Autodesk Inventor part; units mm, degrees
ref_plane "YZ Plane" through (0, 0, 0) normal (1, 0, 0) x (0, 1, 0)
ref_plane "XZ Plane" through (0, 0, 0) normal (0, 1, 0) x (-1, 0, 0)
ref_plane "XY Plane" through (0, 0, 0) normal (0, 0, 1) x (1, 0, 0)
sketch "草圖3" plane through (0, 0, 0) normal (0, 1, 0) x (-1, 0, 0)
  circle A0 centre (0, 0) radius 25
  circle A1 centre (0, 0) radius 70
  line L0 (5, 5) -> (61, 5)
  line L1 (61, 5) -> (61, 32.4)
  line L2 (61, 32.4) -> (5, 32.4)
  line L3 (5, 32.4) -> (5, 5)
  line L4 (19, 33.9) -> (12, 33.9)
  line L5 (12, 33.9) -> (12, 30.9)
  line L6 (12, 30.9) -> (19, 30.9)
  line L7 (19, 30.9) -> (19, 33.9)
  line L8 (54, 33.9) -> (47, 33.9)
  line L9 (47, 33.9) -> (47, 30.9)
  line L10 (47, 30.9) -> (54, 30.9)
  line L11 (54, 30.9) -> (54, 33.9)
  line L12 (61, 18.7) -> (5, 18.7)
  line L13 (19, 3.5) -> (12, 3.5)
  line L14 (12, 3.5) -> (12, 6.5)
  line L15 (12, 6.5) -> (19, 6.5)
  line L16 (19, 6.5) -> (19, 3.5)
  line L17 (54, 3.5) -> (47, 3.5)
  line L18 (47, 3.5) -> (47, 6.5)
  line L19 (47, 6.5) -> (54, 6.5)
  line L20 (54, 6.5) -> (54, 3.5)
  line L21 (0, 0) -> (55, 0)
  line L22 (19.1511, -16.0697) -> (42.1324, -35.3533)
  arc A2 (42.1324, -35.3533) -> (55, 0) centre (0, 0) ccw
  line L23 (0, 0) -> (15.7742, -52.6894)
  arc A3 (-21.7844, -50.5019) -> (15.7742, -52.6894) centre (0, 0) ccw
  line L24 (-9.902, -22.9554) -> (-21.7844, -50.5019)
  line L25 (0, 0) -> (-45.9518, -30.223)
  arc A4 (-54.6281, 6.3851) -> (-45.9518, -30.223) centre (0, 0) ccw
  line L26 (-24.831, 2.9023) -> (-54.6281, 6.3851)
  line L27 (0, 0) -> (-42.1324, 35.3533)
  arc A5 (-9.5506, 54.1644) -> (-42.1324, 35.3533) centre (0, 0) ccw
  line L28 (-4.3412, 24.6202) -> (-9.5506, 54.1644)
  line L29 (17.5, 0) -> (-21.7065, 0)
  line L30 (7.8968, 70) -> (-12.1032, 70)
  line L31 (-12.1032, 70) -> (-12.1032, 0)
  line L32 (-12.1032, 0) -> (7.8968, 0)
  line L33 (7.8968, 0) -> (7.8968, 70)
  point P0 (25, 0)
  point P1 (12, 32.4)
  point P2 (47, 32.4)
  point P3 (12, 5)
  point P4 (47, 5)
  point P5 (0, -70)
  point P6 (-20.8872, -13.7377)
  point P7 (-19.1511, 16.0697)
  point P8 (-4.3412, 24.6202)
  point P9 (25, 0)
  point P10 (-2.1032, 0)
  point P11 (7.1701, -23.9497)
  point P12 (-9.902, -22.9554)
  point P13 (-12.1032, 21.8749)
  point P14 (-12.1032, 33.2534)
  point P15 (-12.1032, 68.9457)
  point P16 (7.8968, 69.5532)
  point P17 (7.8968, 23.7201)
  point P18 (-12.1032, 53.6518)
  point P19 (0, 70)
  point P20 (-12.1032, 10.1558)
  dimension "d19" = 140
  dimension "d30" = 56
  dimension "d31" = 27.4
  dimension "d32" = 5
  dimension "d34" = 3
  dimension "d35" = 7
  dimension "d36" = 3
  dimension "d37" = 7
  dimension "d38" = 7
  dimension "d39" = 7
  dimension "d48" = 50
  dimension "d54" = 36
  dimension "d55" = 55
  dimension "d56" = 40
  dimension "d57" = 0
  dimension "d60" = 220
  dimension "d62" = 20
  dimension "d63" = 70
  dimension "d64" = 53.1032
  dimension "d65" = 30.9
  dimension "d66" = 36
  dimension "d67" = 30.9
  dimension "d68" = 43.5
  dimension "d69" = 61
  dimension "d70" = 30.9
  dimension "d71" = 61
  dimension "d72" = 30.9
  dimension "d73" = 100.9
  dimension "d74" = 69.5505
  dimension "d75" = 7.4077
  dimension "d76" = 80.1511
  dimension "d77" = 46.9697
  dimension "d78" = 82.6506
  dimension "d79" = 18.4
  dimension "d80" = 86
  dimension "d81" = 30.9
extrude "擠出2" add sketch "草圖3" against normal blind 3 contours A0 L23 L21 | L22 A2 L21 A0 L0 L18 L17 L20 L1 L2 L11 L8 L9 L7 L4 L5 L33 A1 L31 A5 L27 L26 A4 L25 L24 A3 L23 | L21 L33 L0 L14 L13 L16 A0 | A0 L25 L23 | L0 L16 L15 L14 L33 L12 A0 | A0 L12 L1 L0 L20 L19 L18 | L25 A0 L27 L31 L29 | L12 L33 A0 | A0 L33 L2 L5 L6 L7 L9 L10 L11 L1 L12 | L16 L13 L14 L0 | L0 L14 L15 L16 | L18 L19 L20 L0 | L0 L20 L17 L18 | L27 A0 L31 | L27 A5 L31 A0 | L5 L4 L7 L2 | L2 L7 L6 L5 | L11 L10 L9 L2 | L2 L9 L8 L11
properties part number "轉盤"
Model file for the job. Use its own axes, mm. A direction names the side the tool comes from. Give positions to 0.01 mm unless a question says otherwise; leave off trailing zeros. Order: outer loops, then holes, each group sorted by start corner. A loop starts at its lowest first (then second) coordinate and runs counter-clockwise, first axis right, second up. Notation, with made-up numbers: (-34, -25.75) - (-8, -25.75) arc R22 ccw to (-8, -10.75) - close; hole circle Ø8 at (17, -24). An arc over 180 degrees is marked (long way). Write item = value, one per line. Start each with the question number.
1. Which spindle directions (+Z, -Z, +X, -X, +Y, -Y) get a long thin tool onto all of the face, cutting with end or side? Do faces 4 (the flat face through (-15, -3, 1)), 5 (the flat face through (-11.412, -1.479, -38.118)), 6 (the flat face through (-7.897, -1, 34)). Say none if no direction does.
2. Two-plate mould, pull along Z, no slides. Class faces 1 (the flat face through (12.103, -1, 35)), 2 (the flat face through (15.76, -1.48, -36.54)), 3 (the flat face through (2, -1, 0)): pulls with the +Z half, pulls with the -Z half, needs draft (parallel to the pull), parting line crosses it, or undercut.
3. Drop flat-ended pins along their axis: P1, Ø0.9, axis at y = -2, z = 29.5, coming from the +X side; P2, Ø0.9, axis at y = -1, z = 45.5, coming from the -X side; P3, Ø1, axis at x = -41.5, y = -0.5, coming from the +Z side. Give the stop position or say it passes through.
4. Cut at C-C, the plane y = -2.5. List the corners of the cut face in (x, z).
5. Cut at D-D, the plane x = -59. List the corners of the cut face in (y, z).
6. Probe line 1 along X through (y, z) = (-1.7, -19); line 2 along X through (y, z) = (-2.4, 39); line 3 along X through (y, z) = (-2.75, 7). List the from-to ranges inside material, lowest first.
7. Cut at B-B, the plane z = 14. List the corners of the cut face in (x, y), and give its area (3 significant figures).
8. Cut at A-A, the plane x = 0. List the corners of the cut face in (y, z), and give its area (3 significant figures).
Taken from the geometry:
q1.face_4 = +Z, -Z, +X, -X, -Y
q1.face_5 = +Y, -Y
q1.face_6 = +Z, +Y, -Y
q2.face_1 = needs draft
q2.face_2 = undercut
q2.face_3 = pulls with the +Z half
q3.P1 = 63.69
q3.P2 = -53.58
q3.P3 = 56.74
q4.outline = (-7.9, 0) - (-7.9, 69.55) arc R70 ccw (long way) to (12.1, 68.95) - (12.1, 0) - close; hole (-55, 0) arc R55 ccw to (-42.13, -35.35) - (-19.15, -16.07) arc R25 cw to (-25, 0) - close; hole (-15.77, -52.69) arc R55 ccw to (21.78, -50.5) - (9.9, -22.96) arc R25 cw to (-7.17, -23.95) - close; hole (20.89, -13.74) - (45.95, -30.22) arc R55 ccw to (54.63, 6.39) - (24.83, 2.9) arc R25 cw to start
q5.outline = (-3, -37.67) - (0, -37.67) - (0, 37.67) - (-3, 37.67) - close
q6.line_1 = -67.37 to -51.61, -22.64 to 28.89, 51.61 to 67.37
q6.line_2 = -58.13 to -7.9, 12.1 to 58.13
q6.line_3 = -69.65 to -7.9, 12.1 to 69.65
q7.outline = (-68.59, -3) - (-7.9, -3) - (-7.9, 0) - (-68.59, 0) - close; (12.1, -3) - (68.59, -3) - (68.59, 0) - (12.1, 0) - close
q7.area = 352 mm²
q8.outline = (-3, -70) - (0, -70) - (0, -55) - (-3, -55) - close; (-3, -25) - (0, -25) - (0, 0) - (-3, 0) - close
q8.area = 120 mm²
